Build history of the part. All positions in model axes, mm. Face numbers are marked on the shaded views. Give positions to 0.01 mm unless a question says otherwise; leave off trailing zeros. Write each loop counter-clockwise with the first axis right and the second up, starting at its lowest first coordinate (ties: lowest second). Pieces come first, ordered by that corner, then holes. Notation, with made-up numbers: (26.5, -3.5) -> (47.5, -3.5) arc R14 ccw to (47.5, 12.5) -> close; hole circle Ø6 at (-33.5, 33). An arc over 180 degrees is marked (long way). Put each result on its own line as item: value. Start each with the question number.
Item 1: Slice it at D-D, the plane z = -11.5. List the corners of the cut face in (x, y).
Item 2: Flat gauge pins, fed straight in: pin 1 Ø5 at (y, z) = (-117.5, 9) entering from -X; pin 2 Ø8 at (y, z) = (-19.5, 8) entering from -X; pin 3 Ø2 at (y, z) = (-46.5, 9.5) entering from -X; pin 4 Ø6 at (x, z) = (11, 6.5) entering from -Y. Where does each tip first touch, or does it go through?
Item 3: Slice it at B-B, the plane x = 7. List the corners of the cut face in (y, z).
Item 4: Slice it at A-A, the plane z = 3. List the corners of the cut face in (x, y) (3 decimals).
Item 5: Two-plate mould, pull along Z, no slides. Class the marked faces 1 and 2: pulls with the +Z half, pulls with the -Z half, needs draft (parallel to the pull), parting line crosses it, or undercut.
Item 6: Slice it at C-C, the plane y = -74. List the corners of the cut face in (x, z), plus the area to 3 significant figures.
Item 7: Drill centre lines: line 1 along X through (y, z) = (-32.5, -4); line 2 along Z through (x, y) = (-6, -29); line 3 along X through (y, z) = (-112.5, -1). Where is each one in solid material? Low to high.
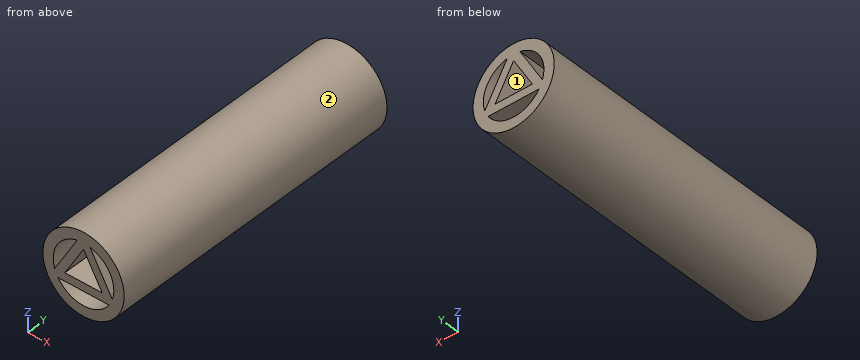
```python
from build123d import *

# Parameters (mm, degrees)
F0_R     = 18.7507393172
F0_W     = 2.8121968498
F0_H     = 2.6235150942
F1_DEPTH = 139.7


# Not quite as in the source:
# - a feature names something its author has since deleted; it is built from what else it names


with BuildPart() as f1:
    # F0 (on Front) → F1 (new body)
    with BuildSketch(Plane.XZ):
        Circle(F0_R)
        with BuildLine():
            ThreePointArc((11.7463163557, -7.5817653145), (0, -13.9806692691), (-11.7463163557, -7.5817653145))
            Line((-11.7463163557, -7.5817653145), (11.7463163557, -7.5817653145))
        make_face(mode=Mode.SUBTRACT)
        with BuildLine():
            ThreePointArc((-13.3049026907, -4.2940281328), (-12.107614749, 6.9903346346), (-2.9337138978, 13.6693977914))
            Line((-2.9337138978, 13.6693977914), (-13.3049026907, -4.2940281328))
        make_face(mode=Mode.SUBTRACT)
        with Locations((-0.1412869315, 14.9811553385)):
            Rectangle(F0_W, F0_H, mode=Mode.SUBTRACT)
        Polygon((-8.6039650607, -3.7717653145), (0, 11.1307393172), (8.6039650607, -3.7717653145), align=None, mode=Mode.SUBTRACT)
        with BuildLine():
            ThreePointArc((2.9337138978, 13.6693977914), (12.107614749, 6.9903346346), (13.3049026907, -4.2940281328))
            Line((13.3049026907, -4.2940281328), (2.9337138978, 13.6693977914))
        make_face(mode=Mode.SUBTRACT)
        with Locations((-0.1412869315, 14.9811553385)):
            Rectangle(F0_W, F0_H)
    extrude(amount=F1_DEPTH)


solid = f1.part
```
Values follow:
1. outline: (-14.81, -139.7) -> (-7.95, -139.7) -> (-7.95, 0) -> (-14.81, 0) -> close; (7.95, -139.7) -> (14.81, -139.7) -> (14.81, 0) -> (7.95, 0) -> close
2. pin 1: x = -17.59
2. pin 2: x = -18.32
2. pin 3: x = -16.71
2. pin 4: y = -139.7
3. outline: (-139.7, -17.4) -> (0, -17.4) -> (0, -12.1) -> (-139.7, -12.1) -> close; (-139.7, -7.58) -> (0, -7.58) -> (0, -3.77) -> (-139.7, -3.77) -> close; (-139.7, -0.99) -> (0, -0.99) -> (0, 6.63) -> (-139.7, 6.63) -> close; (-139.7, 12.1) -> (0, 12.1) -> (0, 17.4) -> (-139.7, 17.4) -> close
4. outline: (-18.509, -139.7) -> (-13.655, -139.7) -> (-13.655, 0) -> (-18.509, 0) -> close; (-9.094, -139.7) -> (-4.694, -139.7) -> (-4.694, 0) -> (-9.094, 0) -> close; (4.694, -139.7) -> (9.094, -139.7) -> (9.094, 0) -> (4.694, 0) -> close; (13.655, -139.7) -> (18.509, -139.7) -> (18.509, 0) -> (13.655, 0) -> close
5. face 1: undercut
5. face 2: parting line crosses it
6. outline: circle Ø37.5 at (0, 0); hole (-13.3, -4.29) -> (-2.93, 13.67) arc R13.98 ccw to start; hole (-11.75, -7.58) arc R13.98 ccw to (11.75, -7.58) -> close; hole (-8.6, -3.77) -> (8.6, -3.77) -> (0, 11.13) -> close; hole (2.93, 13.67) -> (13.3, -4.29) arc R13.98 ccw to start
6. area: 738 mm2
7. line 1: -18.32 to -13.4, -13.14 to 13.14, 13.4 to 18.32
7. line 2: -17.76 to -12.63, -7.58 to -3.77, 0.74 to 8.36, 12.63 to 17.76
7. line 3: -18.72 to -13.94, -11.4 to -7, 7 to 11.4, 13.94 to 18.72
